Verification items for the finished model (mm, model axes). Give positions to 0.01 mm unless a question says otherwise; leave off trailing zeros. Loops run counter-clockwise (first coordinate to the right, second up) from the corner with the lowest first, then second, coordinate; pieces in that order, holes last. Notation, with made-up numbers: (45.5, 20.5) - (51.5, 20.5) arc R22 cw to (51.5, 55.5) - close; hole circle Ø6 at (16.5, 31). An arc over 180 degrees is marked (long way). One line per question, with ' | ' between items. Start each with the question number.
1. Section check C-C, the plane x = 10. Enter the section's corners in (y, z), then the cut area to 3 significant figures.
2. Mould release check, pull along Z, two halves, no side actions. Record for faces 1 (the face through (10.763, 0.094, 0.336)), 2 (the face through (3, 0, 26)), 3 (the face through (-13, 0, 0)), 4 (the face through (3, 0, -26)): +Z half, -Z half, draft (parallel to the pull), parting line (faces both ways), or undercut.
3. Depth check by flat-ended pin: pin 1 Ø10 at (x, z) = (9.5, -16) entering from +Y. Enter the tip coordinate at first touch or a pass-through.
4. Thickness scan on line 1 along Z through (x, y) = (10.25, 0.45); line 2 along Y through (x, z) = (8.5, -21.5); line 3 along Y through (x, z) = (9.25, -23). Record the ranges inside material, lowest first. Write a range as from..to.
5. Section check B-B, the plane y = 0.1. Enter the section's corners in (x, z).
6. Section check A-A, the plane z = -13. Enter the section's corners in (x, y), then the cut area to 3 significant figures.
7. Section check D-D, the plane z = -20.5. Enter the section's corners in (x, y), then the cut area to 3 significant figures.
from build123d import *

# Parameters (mm, degrees)
BOSS_EXTRUDE1_DEPTH = 0.5
CUT_EXTRUDE4_DEPTH  = 24


with BuildPart() as part:
    # Sketch1 → Boss-Extrude1 (new body, symmetric)
    with BuildSketch(Plane(origin=(0, 0, 0), x_dir=(1, 0, 0), z_dir=(0, 1, 0))):
        with BuildLine():
            Line((-7, -26), (13, -26))
            Line((13, -26), (13, 26))
            Line((13, 26), (-7, 26))
            ThreePointArc((-7, 26), (-11.242640687, 24.242640687), (-13, 20))
            Line((-13, 20), (-13, -20))
            ThreePointArc((-13, -20), (-11.242640687, -24.242640687), (-7, -26))
        make_face()
    extrude(amount=BOSS_EXTRUDE1_DEPTH, both=True)

    # Sketch2 → Cut-Extrude4 (cut, symmetric)
    with BuildSketch(Plane.XY):
        Polygon((13, -0.3), (8.462974544, 0.5), (13, 0.5), align=None)
    extrude(amount=CUT_EXTRUDE4_DEPTH, both=True, mode=Mode.SUBTRACT)


solid = part.part
Results list:
1) outline: (-0.5, -26) - (0.5, -26) - (0.5, -24) - (0.23, -24) - (0.23, 24) - (0.5, 24) - (0.5, 26) - (-0.5, 26) - close | area: 39.0 mm²
2) face 1: undercut | face 2: +Z half | face 3: draft | face 4: -Z half
3) pin 1: y = 0.5
4) line 1: -26..-24, 24..26 | line 2: -0.5..0.49 | line 3: -0.5..0.36
5) outline: (-13, -20) arc R6 ccw to (-7, -26) - (13, -26) - (13, -24) - (10.73, -24) - (10.73, 24) - (13, 24) - (13, 26) - (-7, 26) arc R6 ccw to (-13, 20) - close
6) outline: (-13, -0.5) - (13, -0.5) - (13, -0.3) - (8.46, 0.5) - (-13, 0.5) - close | area: 24.2 mm²
7) outline: (-12.98, -0.5) - (13, -0.5) - (13, -0.3) - (8.46, 0.5) - (-12.98, 0.5) - close | area: 24.2 mm²
